from build123d import *

# Parameters (mm, degrees)
PAD_DEPTH = 10


with BuildPart() as part:
    # Sketch → Pad (new body)
    with BuildSketch(Plane(origin=(0, 0, 0), x_dir=(0.866025, 0.5, 0), z_dir=(0, 0, 1))):
        with BuildLine():
            Line((290, 0), (289.7129, 0.0174))
            Line((289.7129, 0.0174), (288.8574, 0.0696))
            Line((288.8574, 0.0696), (287.4306, 0.1769))
            Line((287.4306, 0.1769), (285.4441, 0.3509))
            Line((285.4441, 0.3509), (282.9037, 0.6003))
            Line((282.9037, 0.6003), (279.8181, 0.9251))
            Line((279.8181, 0.9251), (276.1989, 1.3224))
            Line((276.1989, 1.3224), (272.0635, 1.7893))
            Line((272.0635, 1.7893), (267.4264, 2.3229))
            Line((267.4264, 2.3229), (262.3079, 2.9261))
            Line((262.3079, 2.9261), (256.7254, 3.6076))
            Line((256.7254, 3.6076), (250.6992, 4.3587))
            Line((250.6992, 4.3587), (244.2583, 5.1852))
            Line((244.2583, 5.1852), (237.4259, 6.0784))
            Line((237.4259, 6.0784), (230.2281, 7.0383))
            Line((230.2281, 7.0383), (230.2281, 40.028069))
            Line((230.2281, 40.028069), (201.90651, 39.515951))
            ThreePointArc((172.217343, 14.637652), (187.660006, 26.363067), (201.90651, 39.515951))
            Line((172.217343, 14.637652), (163.1743, 16.2081))
            Line((163.1743, 16.2081), (154.106, 17.371))
            Line((154.106, 17.371), (145, 18.4817))
            Line((145, 18.4817), (135.8969, 19.5199))
            Line((135.8969, 19.5199), (126.8257, 20.4682))
            Line((126.8257, 20.4682), (117.8299, 21.3034))
            Line((117.8299, 21.3034), (108.9414, 22.0023))
            Line((108.9414, 22.0023), (100.1921, 22.5446))
            Line((100.1921, 22.5446), (91.6226, 22.9129))
            Line((91.6226, 22.9129), (83.2619, 23.0898))
            Line((83.2619, 23.0898), (75.1448, 23.0608))
            Line((75.1448, 23.0608), (67.3061, 22.8201))
            Line((67.3061, 22.8201), (59.7719, 22.3561))
            Line((59.7719, 22.3561), (52.5741, 21.6717))
            Line((52.5741, 21.6717), (45.7417, 20.7698))
            Line((45.7417, 20.7698), (39.3008, 19.662))
            Line((39.3008, 19.662), (33.2746, 18.3628))
            Line((33.2746, 18.3628), (27.6921, 16.8896))
            Line((27.6921, 16.8896), (22.5736, 15.2714))
            Line((22.5736, 15.2714), (17.9365, 13.5314))
            Line((17.9365, 13.5314), (13.8011, 11.7015))
            Line((13.8011, 11.7015), (10.1819, 9.8165))
            Line((10.1819, 9.8165), (7.0963, 7.9112))
            Line((7.0963, 7.9112), (4.5559, 6.0378))
            Line((4.5559, 6.0378), (2.5694, 4.263))
            Line((2.5694, 4.263), (1.1426, 2.6535))
            Line((1.1426, 2.6535), (0.2871, 1.2383))
            Line((0.2871, 1.2383), (0, 0))
            Line((0, 0), (0.2871, -1.131))
            Line((0.2871, -1.131), (1.1426, -2.2243))
            Line((1.1426, -2.2243), (2.5694, -3.3176))
            Line((2.5694, -3.3176), (4.5559, -4.3964))
            Line((4.5559, -4.3964), (7.0963, -5.4201))
            Line((38.675534, -31.593528), (7.0963, -5.4201))
            Line((38.675534, -31.593528), (232.520951, -31.593528))
            Line((232.520951, -31.593528), (244.2583, -4.8227))
            Line((244.2583, -4.8227), (250.6992, -4.1267))
            Line((250.6992, -4.1267), (256.7254, -3.4626))
            Line((256.7254, -3.4626), (262.3079, -2.842))
            Line((262.3079, -2.842), (267.4264, -2.2765))
            Line((267.4264, -2.2765), (272.0635, -1.7661))
            Line((272.0635, -1.7661), (276.1989, -1.3137))
            Line((276.1989, -1.3137), (279.8181, -0.9222))
            Line((279.8181, -0.9222), (282.9037, -0.5974))
            Line((282.9037, -0.5974), (285.4441, -0.3509))
            Line((285.4441, -0.3509), (287.4306, -0.1769))
            Line((287.4306, -0.1769), (288.8574, -0.0696))
            Line((288.8574, -0.0696), (289.7129, -0.0174))
            Line((289.7129, -0.0174), (290, 0))
        make_face()
    extrude(amount=PAD_DEPTH)


solid = part.part
Here's how the part is built. I have some questions about the finished solid (model axes, mm). A direction names the side the tool comes from. Round coordinates to 2 decimals unless told otherwise and drop trailing zeros. Write each loop counter-clockwise with the first axis right and the second up, starting at its lowest first coordinate (ties: lowest second). Pieces come first, ordered by that corner, then holes. Notation, with made-up numbers: (71.25, -34.75) -> (114.25, -34.75) arc R12 ccw to (114.25, -17.75) -> close; hole circle Ø9 at (-19, 28.5). An arc over 180 degrees is marked (long way). One line per item, written item: value.
1) If I drill on line 1 (X direction, y = 125, z = 4); line 2 (X direction, y = 135.5, z = 2.75); line 3 (Y direction, x = 34, z = 3.75), over which ranges is the centre line in solid material (lowest first)? Write a range as [from, to].
Filled sheet:
line 1: x = [152.17, 193.68], [205.04, 223.57]
line 2: x = [155.64, 187.61], [229.91, 237.86]
line 3: y = [-5.42, 44.52]
2) Suppose I cut it at B-B on x = 137.5. List the corners of the cut face in (y, z) for me, plus the area to 3 significant figures.
Filled sheet:
outline: (42.9, 0) -> (97.2, 0) -> (97.2, 10) -> (42.9, 10) -> close
area: 543 mm2
3) I'm going to push flat-ended pins straight in: pin 1 Ø4 at (y, z) = (24, 1) entering from -X; pin 2 Ø4 at (x, z) = (154, 5.5) entering from -Y; pin 3 Ø4 at (y, z) = (30.5, 8.5) entering from +X. Where does each tip first touch, or does it pass through?
Filled sheet:
pin 1: stops at x = 9.85
pin 2: stops at y = 51.28
pin 3: stops at x = 119.48
4) We'd pull the mould along Y, two halves only. Please class faces 3 (the face through (215.58, 103.22, 4.93)), 4 (the face through (228.1, 134.72, 4.93)), 5 (the face through (125, 69, 0)), 6 (the face through (29.356, -4.633, 4.93)): released by +Y, released by -Y, zero draft, split by the parting line, or undercut.
Filled sheet:
face 3: undercut
face 4: released by +Y
face 5: zero draft
face 6: released by -Y
5) Suppose I cut it at A-A on y = 107. List the corners of the cut face in (x, z) for me, plus the area to 3 significant figures.
Filled sheet:
outline: (145.53, 0) -> (215.16, 0) -> (215.16, 10) -> (145.53, 10) -> close
area: 696 mm2
6) For faces 1 (the face through (32, 42.986, 4.93)), 2 (the face through (217.769, 130.322, 4.93)), which set-ups out of +Z, -Z, +X, -X, +Y, -Y let a thin tool reach every point of the face, with its end or its side?
Filled sheet:
face 1: +Z, -Z, -X, +Y
face 2: +Z, -Z, +Y
